Source: three-view drawing plus pictorial views. Frame: mm from the lowest corner of the part. A direction names the side the tool comes from. Give positions to 0.01 mm unless a question says otherwise; leave off trailing zeros. Order: outer loops, then holes, each group sorted by start corner. A loop starts at its lowest first (then second) coordinate and runs counter-clockwise, first axis right, second up.
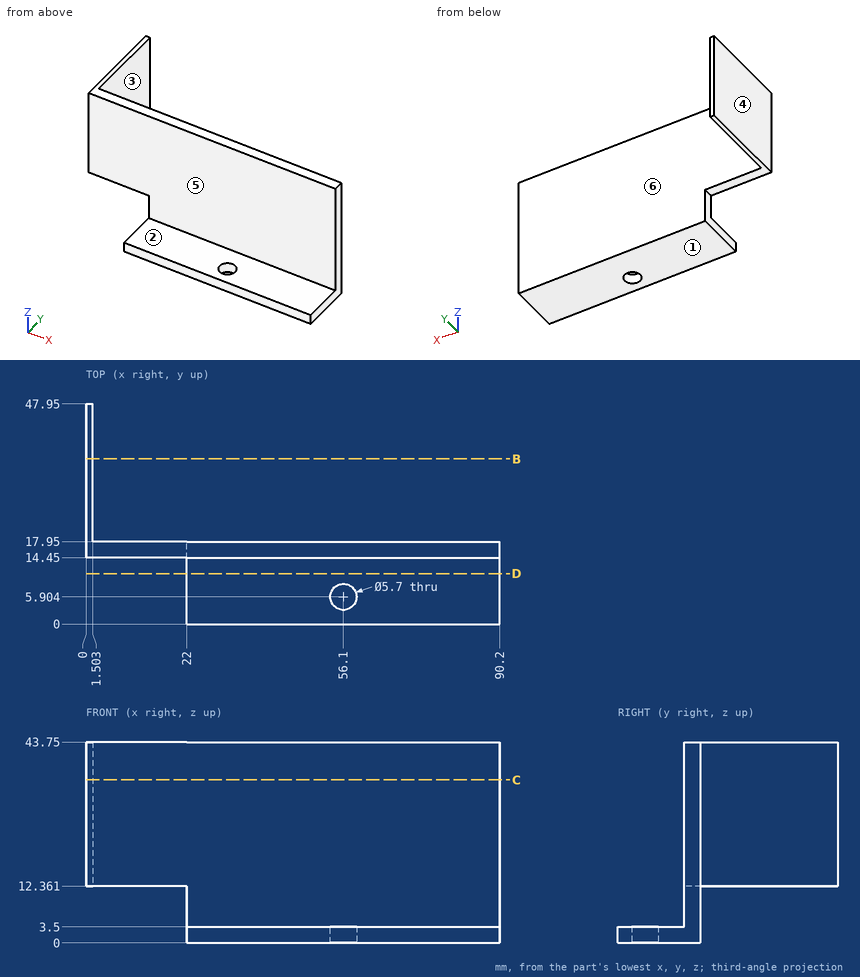
1) Pull-direction query (Y, two-part tool) for the marked faces 4, 5 and 6; classes: +Y half, -Y half, draft (parallel to the pull), parting line (faces both ways), or undercut.
Checks:
face 4: draft
face 5: -Y half
face 6: +Y half
2) Reachability of the marked faces 1, 2 and 3 from +Z, -Z, +X, -X, +Y, -Y: full face, straight path, thin tool, end or side. Return the list, or none.
Checks:
face 1: -Z, +X, -X, +Y, -Y
face 2: +Z, +X, -X, -Y
face 3: +Z, -Z, +X, +Y
3) Ray query, L1, parallel to Y at x = 56, z = 2; L2, parallel to Z at x = 70, y = 9; L3, parallel to X at y = 24, z = 38.5. Return the intervals inside material, ascending.
Checks:
L1: y = 0 to 3.06, 8.75 to 17.95
L2: z = 0 to 3.5
L3: x = 0 to 1.5
4) Section query D-D on y = 11. Output: boundary loops of the cut face in (x, z).
Checks:
outline: (22, 0) - (90.2, 0) - (90.2, 3.5) - (22, 3.5) - close
5) First-contact query: pin 1 Ø1 at (y, z) = (41, 36) entering from +X; pin 2 Ø5 at (x, z) = (43, 17.5) entering from -Y; pin 3 Ø5 at (y, z) = (30.5, 28) entering from -X; pin 4 Ø1.5 at (x, z) = (70.5, 34.5) entering from +Y. Flat tips, straight axial feed; report the tip coordinate or a pass-through.
Checks:
pin 1: stops at x = 1.5
pin 2: stops at y = 14.45
pin 3: stops at x = 0
pin 4: stops at y = 17.95
6) Section query C-C on z = 35.5. Output: boundary loops of the cut face in (x, y).
Checks:
outline: (0, 14.45) - (90.2, 14.45) - (90.2, 17.95) - (1.5, 17.95) - (1.5, 47.95) - (0, 47.95) - close
7) Section query B-B on y = 36. Output: boundary loops of the cut face in (x, z).
Checks:
outline: (0, 12.36) - (1.5, 12.36) - (1.5, 43.75) - (0, 43.75) - close
